```python
from build123d import *

# Parameters (mm, degrees)
SKETCH1_W           = 71
SKETCH1_H           = 71
SKETCH1_R           = 3
SKETCH1_R_2         = 28
BOSS_EXTRUDE1_DEPTH = 10
SKETCH2_W           = 71
SKETCH2_H           = 71
SKETCH2_R           = 28
REVOLVE1_ANGLE      = 30
LPATTERN1_COUNT     = 3
LPATTERN1_PITCH     = 70
SKETCH3_W           = 20
SKETCH3_H           = 71
BOSS_EXTRUDE2_DEPTH = 10
SKETCH4_R           = 4
CUT_EXTRUDE1_DEPTH  = 10


with BuildPart() as part:
    # Sketch1 → Boss-Extrude1 (new body)
    with BuildSketch(Plane(origin=(0, 0, 0), x_dir=(1, 0, 0), z_dir=(0, 1, 0))):
        with Locations((-15.992227979, 8.554404145)):
            Rectangle(SKETCH1_W, SKETCH1_H)
        with Locations((-43.492227979, 37.054404145)):
            Circle(SKETCH1_R, mode=Mode.SUBTRACT)
        with Locations((12.507772021, 37.054404145)):
            Circle(SKETCH1_R, mode=Mode.SUBTRACT)
        with Locations((12.507772021, -18.945595855)):
            Circle(SKETCH1_R, mode=Mode.SUBTRACT)
        with Locations((-43.492227979, -18.945595855)):
            Circle(SKETCH1_R, mode=Mode.SUBTRACT)
        with Locations((-15.992227979, 8.554404145)):
            Circle(SKETCH1_R_2, mode=Mode.SUBTRACT)
    boss_extrude1 = extrude(amount=BOSS_EXTRUDE1_DEPTH)

    # Sketch2 → Revolve1 (revolve)
    with BuildSketch(Plane.XZ):
        with Locations((-15.992227979, -8.554404145)):
            Rectangle(SKETCH2_W, SKETCH2_H)
        with Locations((-15.992227979, -8.554404145)):
            Circle(SKETCH2_R, mode=Mode.SUBTRACT)
    revolve1 = revolve(axis=Axis((19.507772021, 0, 26.945595855), (-1, 0, 0)), revolution_arc=REVOLVE1_ANGLE)

    # LPattern1: Boss-Extrude1, Revolve1 ×3
    with Locations(*[(i * LPATTERN1_PITCH, 0, 0) for i in range(1, LPATTERN1_COUNT)]):
        add(boss_extrude1)
        add(revolve1)

    # Sketch3 → Boss-Extrude2 (add)
    with BuildSketch(Plane(origin=(0, -11.667785265, 6.736398964), x_dir=(1, 0, 0), z_dir=(0, -0.866025404, 0.5))):
        with Locations((-61.492227979, -12.16442947)):
            Rectangle(SKETCH3_W, SKETCH3_H)
    extrude(amount=-BOSS_EXTRUDE2_DEPTH)

    # Sketch4 → Cut-Extrude1 (cut)
    with BuildSketch(Plane(origin=(0, -11.667785265, 6.736398964), x_dir=(1, 0, 0), z_dir=(0, -0.866025404, 0.5))):
        with Locations((-63.492227979, 15.33557053)):
            Circle(SKETCH4_R)
        with Locations((-63.492227979, -39.66442947)):
            Circle(SKETCH4_R)
    extrude(amount=-CUT_EXTRUDE1_DEPTH, mode=Mode.SUBTRACT)


solid = part.part
```
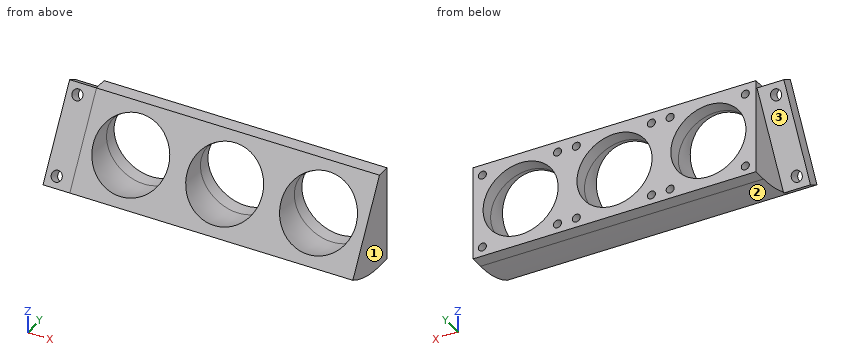
Build history of the part. All positions in model axes, mm. Face numbers are marked on the shaded views. A direction names the side the tool comes from. Coordinates: 2 decimals unless noted, no trailing zeros. Order: outer loops, then holes, each group sorted by start corner. A loop starts at its lowest first (then second) coordinate and runs counter-clockwise, first axis right, second up. Notation, with made-up numbers: (76.25, 10.25) -> (115.25, 10.25) arc R13 cw to (115.25, 17.25) -> close; hole circle Ø1 at (36.5, -32). An arc over 180 degrees is marked (long way). Answer in a Markdown table with one row per item. Add a question column.
Q1. Drop flat-ended pins along their axis: pin 1 (12 mm diameter, centred on x = 22, z = 12, fed in from -Y); pin 2 (5.5 mm diameter, centred on x = 152.51, z = 18.95, fed in from -Y); pin 3 (1.8 mm diameter, centred on x = 153, z = -36.5, fed in from +Y). Give the stop position or say it passes through.
Q2. Band-saw the part on C-C, the plane x = 18. List the corners of the cut face in (y, z).
Q3. Which spindle directions (+Z, -Z, +X, -X, +Y, -Y) get a long thin tool onto all of the face, cutting with end or side? Do the marked faces 1, 2 and 3. Say none if no direction does.
Q4. Wall check: line 1 along X through (y, z) = (-7, -1.5); line 2 along X through (y, z) = (-28, -23); line 3 along X through (y, z) = (-14.5, -36.5). Give the ranges that are in metal, low to high. Write a range as [from, to].
Q5. Band-saw the part on B-B, the plane z = 8.5. Give the number of separate pieces and of enclosed holes in the cut face, then the cut area to 3 significant figures.
Q6. Band-saw the part on A-A, the plane x = -20.5. List the corners of the cut face in (y, z).
Answers follow:
| question | item | result |
|---|---|---|
| 1 | pin 1 | y = -12.09 |
| 1 | pin 2 | y = -6.2 |
| 1 | pin 3 | y = 0 |
| 2 | outline | (-35.5, -34.54) arc R71 ccw to (0, -44.05) -> (10, -44.05) -> (10, 26.95) -> (0, 26.95) -> close |
| 3 | face 1 | +Z, -Z, +X, +Y, -Y |
| 3 | face 2 | -Z, +X, -Y |
| 3 | face 3 | -Z, -X, +Y |
| 4 | line 1 | [-71.49, -43.3], [11.31, 26.7], [81.31, 96.7], [151.31, 159.51] |
| 4 | line 2 | [-71.49, -33.61], [1.63, 36.39], [71.63, 106.39], [141.63, 159.51] |
| 4 | line 3 | [-51.49, 159.51] |
| 5 | separate pieces | 4 |
| 5 | enclosed holes | 0 |
| 5 | area | 1,790 mm^2 |
| 6 | outline | (-35.5, -34.54) arc R71 ccw to (0, -44.05) -> (10, -44.05) -> (10, -36.19) -> (0, -36.19) arc R63.13 cw to (-31.57, -27.73) -> close; (-3.93, 20.13) arc R7.87 ccw to (0, 19.08) -> (10, 19.08) -> (10, 26.95) -> (0, 26.95) -> close |
